Here's the drawing with two shaded views (mm, measured from the low corner). I have some questions. Round coordinates to 2 decimals unless told otherwise and drop trailing zeros. Loops run counter-clockwise (first coordinate to the right, second up) from the corner with the lowest first, then second, coordinate; pieces in that order, holes last. Notation, with made-up numbers: (47, -38) -> (93, -38) arc R7 ccw to (93, -33) -> close; hole circle Ø7 at (22.25, 52.25). An arc over 180 degrees is marked (long way). Use a Markdown table: item, result.
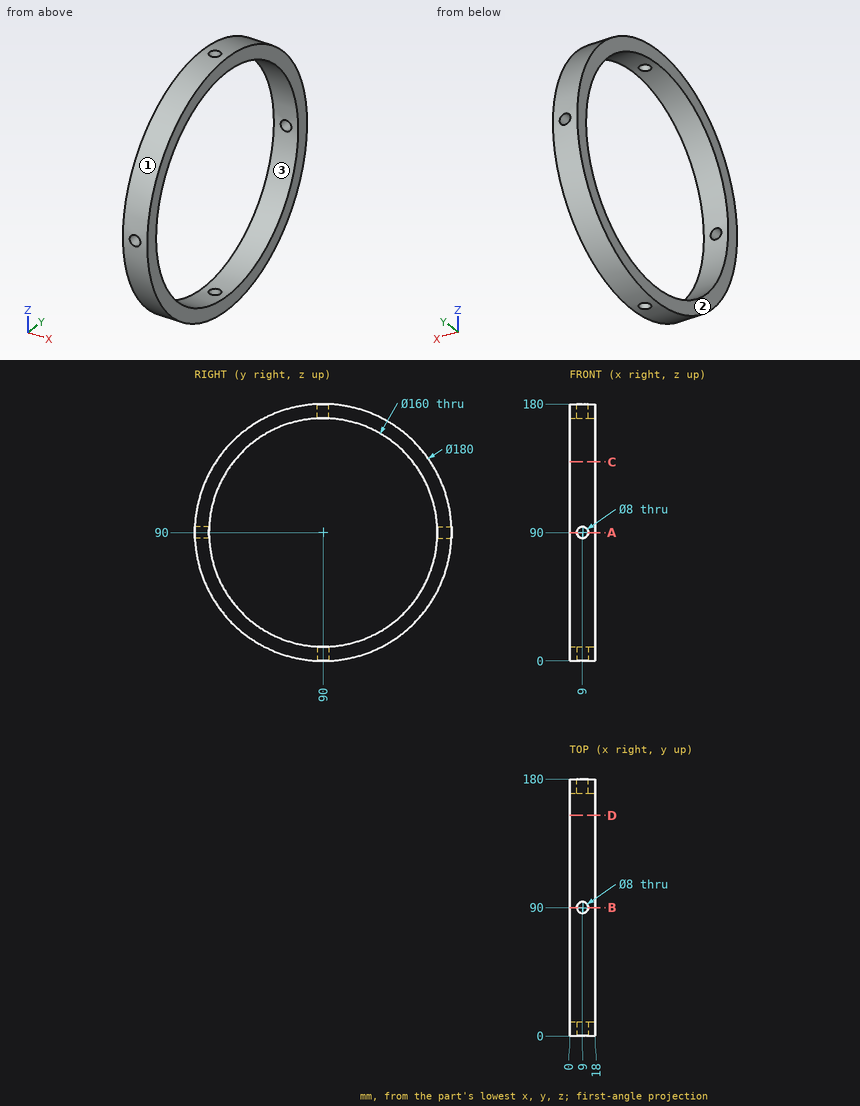
1. I want a section at A-A (z = 90). Please give me the cut outline in (x, y), plus the area to 3 significant figures.
Answer sheet:
| item | result |
|---|---|
| outline | (0, 0) -> (5, 0) -> (5, 10) -> (0, 10) -> close; (0, 170) -> (5, 170) -> (5, 180) -> (0, 180) -> close; (13, 0) -> (18, 0) -> (18, 10) -> (13, 10) -> close; (13, 170) -> (18, 170) -> (18, 180) -> (13, 180) -> close |
| area | 200 mm² |
2. I want a section at D-D (y = 154.5). Please give me the cut outline in (x, z).
Answer sheet:
| item | result |
|---|---|
| outline | (0, 27.23) -> (18, 27.23) -> (18, 42.67) -> (0, 42.67) -> close; (0, 137.33) -> (18, 137.33) -> (18, 152.77) -> (0, 152.77) -> close |
3. Will these pins go through, and if not, where does the flat tip stop? pin 1 Ø9 at (x, y) = (9, 90) entering from -Z; pin 2 Ø8 at (x, y) = (8.5, 62.5) entering from -Z; pin 3 Ø1 at (x, y) = (12.5, 99) entering from +Z; pin 4 Ø5 at (x, z) = (12, 123.5) entering from +Y.
Answer sheet:
| item | result |
|---|---|
| pin 1 | stops at z = 0 |
| pin 2 | stops at z = 3.12 |
| pin 3 | stops at z = 179.6 |
| pin 4 | stops at y = 174.49 |
4. If we mould it in two halves opening along Y, with no side actions, what happens to the marked faces 1, 2 and 3? For each: +Y half, -Y half, draft (parallel to the pull), parting line (faces both ways), or undercut.
Answer sheet:
| item | result |
|---|---|
| face 1 | parting line |
| face 2 | draft |
| face 3 | undercut |
5. I need wall thicknesses on line 1 (X direction, y = 176, z = 90); line 2 (Z direction, x = 7.5, y = 54); line 3 (Z direction, x = 3, y = 114). Which ranges of each line are inside material? Lowest first, please.
Answer sheet:
| item | result |
|---|---|
| line 1 | x = 0 to 5, 13 to 18 |
| line 2 | z = 7.51 to 18.56, 161.44 to 172.49 |
| line 3 | z = 3.26 to 13.68, 166.32 to 176.74 |
6. I want a section at C-C (z = 139.5). Please give me the cut outline in (x, y), plus the area to 3 significant figures.
Answer sheet:
| item | result |
|---|---|
| outline | (0, 14.84) -> (18, 14.84) -> (18, 27.15) -> (0, 27.15) -> close; (0, 152.85) -> (18, 152.85) -> (18, 165.16) -> (0, 165.16) -> close |
| area | 443 mm² |
